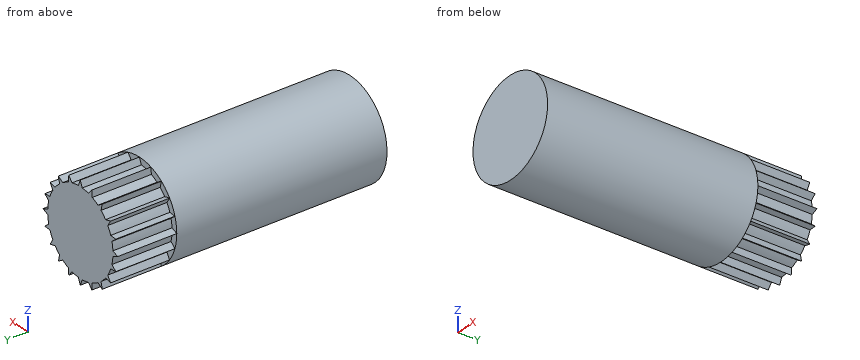
from build123d import *

# Parameters (mm, degrees)
SKETCH1_R           = 4.86
BOSS_EXTRUDE1_DEPTH = 21.336
BOSS_EXTRUDE2_DEPTH = 6


with BuildPart() as part:
    # Sketch1 → Boss-Extrude1 (new body)
    with BuildSketch(Plane(origin=(0, 0, 0), x_dir=(1, 0, 0), z_dir=(0, 1, 0))):
        with Locations(Location((0, 0, 0), (0, 0, 270))):
            Circle(SKETCH1_R)
    extrude(amount=BOSS_EXTRUDE1_DEPTH)

    # Sketch2 → Boss-Extrude2 (add)
    with BuildSketch(Plane(origin=(0, 21.336, 0), x_dir=(1, 0, 0), z_dir=(0, 1, 0))):
        with BuildLine():
            Line((0, 4.86), (0.250754017, 4.242596189))
            ThreePointArc((0.250754017, 4.242596189), (0.664846476, 4.197675448), (1.072553081, 4.112436004))
            Line((1.072553081, 4.112436004), (1.501822593, 4.622134669))
            Line((1.501822593, 4.622134669), (1.549515564, 3.957461499))
            ThreePointArc((1.549515564, 3.957461499), (1.929459624, 3.786777728), (2.29087121, 3.57972193))
            Line((2.29087121, 3.57972193), (2.856636326, 3.931822593))
            Line((2.856636326, 3.931822593), (2.696599732, 3.284942904))
            ThreePointArc((2.696599732, 3.284942904), (3.00520382, 3.00520382), (3.284942904, 2.696599732))
            Line((3.284942904, 2.696599732), (3.931822593, 2.856636326))
            Line((3.931822593, 2.856636326), (3.57972193, 2.29087121))
            ThreePointArc((3.57972193, 2.29087121), (3.786777728, 1.929459624), (3.957461499, 1.549515564))
            Line((3.957461499, 1.549515564), (4.622134669, 1.501822593))
            Line((4.622134669, 1.501822593), (4.112436004, 1.072553081))
            ThreePointArc((4.112436004, 1.072553081), (4.197675448, 0.664846476), (4.242596189, 0.250754017))
            Line((4.242596189, 0.250754017), (4.86, 0))
            Line((4.86, 0), (4.242596189, -0.250754017))
            ThreePointArc((4.242596189, -0.250754017), (4.197675448, -0.664846476), (4.112436004, -1.072553081))
            Line((4.112436004, -1.072553081), (4.622134669, -1.501822593))
            Line((4.622134669, -1.501822593), (3.957461499, -1.549515564))
            ThreePointArc((3.957461499, -1.549515564), (3.786777728, -1.929459624), (3.57972193, -2.29087121))
            Line((3.57972193, -2.29087121), (3.931822593, -2.856636326))
            Line((3.931822593, -2.856636326), (3.284942904, -2.696599732))
            ThreePointArc((3.284942904, -2.696599732), (3.00520382, -3.00520382), (2.696599732, -3.284942904))
            Line((2.696599732, -3.284942904), (2.856636326, -3.931822593))
            Line((2.856636326, -3.931822593), (2.29087121, -3.57972193))
            ThreePointArc((2.29087121, -3.57972193), (1.929459624, -3.786777728), (1.549515564, -3.957461499))
            Line((1.549515564, -3.957461499), (1.501822593, -4.622134669))
            Line((1.501822593, -4.622134669), (1.072553081, -4.112436004))
            ThreePointArc((1.072553081, -4.112436004), (0.664846476, -4.197675448), (0.250754017, -4.242596189))
            Line((0.250754017, -4.242596189), (0, -4.86))
            Line((0, -4.86), (-0.250754017, -4.242596189))
            ThreePointArc((-0.250754017, -4.242596189), (-0.664846476, -4.197675448), (-1.072553081, -4.112436004))
            Line((-1.072553081, -4.112436004), (-1.501822593, -4.622134669))
            Line((-1.501822593, -4.622134669), (-1.549515564, -3.957461499))
            ThreePointArc((-1.549515564, -3.957461499), (-1.929459624, -3.786777728), (-2.29087121, -3.57972193))
            Line((-2.29087121, -3.57972193), (-2.856636326, -3.931822593))
            Line((-2.856636326, -3.931822593), (-2.696599732, -3.284942904))
            ThreePointArc((-2.696599732, -3.284942904), (-3.00520382, -3.00520382), (-3.284942904, -2.696599732))
            Line((-3.284942904, -2.696599732), (-3.931822593, -2.856636326))
            Line((-3.931822593, -2.856636326), (-3.57972193, -2.29087121))
            ThreePointArc((-3.57972193, -2.29087121), (-3.786777728, -1.929459624), (-3.957461499, -1.549515564))
            Line((-3.957461499, -1.549515564), (-4.622134669, -1.501822593))
            Line((-4.622134669, -1.501822593), (-4.112436004, -1.072553081))
            ThreePointArc((-4.112436004, -1.072553081), (-4.197675448, -0.664846476), (-4.242596189, -0.250754017))
            Line((-4.242596189, -0.250754017), (-4.86, 0))
            Line((-4.86, 0), (-4.242596189, 0.250754017))
            ThreePointArc((-4.242596189, 0.250754017), (-4.197675448, 0.664846476), (-4.112436004, 1.072553081))
            Line((-4.112436004, 1.072553081), (-4.622134669, 1.501822593))
            Line((-4.622134669, 1.501822593), (-3.957461499, 1.549515564))
            ThreePointArc((-3.957461499, 1.549515564), (-3.786777728, 1.929459624), (-3.57972193, 2.29087121))
            Line((-3.57972193, 2.29087121), (-3.931822593, 2.856636326))
            Line((-3.931822593, 2.856636326), (-3.284942904, 2.696599732))
            ThreePointArc((-3.284942904, 2.696599732), (-3.00520382, 3.00520382), (-2.696599732, 3.284942904))
            Line((-2.696599732, 3.284942904), (-2.856636326, 3.931822593))
            Line((-2.856636326, 3.931822593), (-2.29087121, 3.57972193))
            ThreePointArc((-2.29087121, 3.57972193), (-1.929459624, 3.786777728), (-1.549515564, 3.957461499))
            Line((-1.549515564, 3.957461499), (-1.501822593, 4.622134669))
            Line((-1.501822593, 4.622134669), (-1.072553081, 4.112436004))
            ThreePointArc((-1.072553081, 4.112436004), (-0.664846476, 4.197675448), (-0.250754017, 4.242596189))
            Line((-0.250754017, 4.242596189), (0, 4.86))
        make_face()
    extrude(amount=BOSS_EXTRUDE2_DEPTH)


solid = part.part
Could you check a few things on this model? Use its own coordinates, in mm. Round coordinates to 2 decimals unless told otherwise and drop trailing zeros. Write each loop counter-clockwise with the first axis right and the second up, starting at its lowest first coordinate (ties: lowest second). Pieces come first, ordered by that corner, then holes. Notation, with made-up numbers: (7.25, 30) -> (46.25, 30) arc R8 cw to (46.25, 42) -> close; hole circle Ø8 at (16, 5). An arc over 180 degrees is marked (long way). Use a Markdown table: item, result.
1. If we section it at C-C (z = -0.5): List the corners of the cut face in (x, y) for me.
Answer key:
| item | result |
|---|---|
| outline | (-4.83, 0) -> (4.83, 0) -> (4.83, 21.34) -> (4.22, 21.34) -> (4.22, 27.34) -> (-4.22, 27.34) -> (-4.22, 21.34) -> (-4.83, 21.34) -> close |
2. If we section it at B-B (y = 13.25): List the corners of the cut face in (x, z) for me.
Answer key:
| item | result |
|---|---|
| outline | circle Ø9.72 at (0, 0) |
3. Please list where these lines run through material, in increasing order: probe 1 along X at (y, z) = (6.5, 0.25); probe 2 along Y at (x, z) = (-2, 4); probe 3 along Z at (x, y) = (1.75, 21.75).
Answer key:
| item | result |
|---|---|
| probe 1 | x = -4.85 to 4.85 |
| probe 2 | y = 0 to 21.34 |
| probe 3 | z = -3.87 to 3.87 |
4. If we section it at A-A (z = 0.75): List the corners of the cut face in (x, y) for me, then the cut area to 3 significant figures.
Answer key:
| item | result |
|---|---|
| outline | (-4.8, 0) -> (4.8, 0) -> (4.8, 21.34) -> (4.18, 21.34) -> (4.18, 27.34) -> (-4.18, 27.34) -> (-4.18, 21.34) -> (-4.8, 21.34) -> close |
| area | 255 mm^2 |
5. For pin 1 Ø1 at (y, z) = (6, -3.5) entering from +X; pin 2 Ø3 at (y, z) = (6.5, 3) entering from -X; pin 3 Ø1.5 at (x, z) = (3.5, -3) entering from -Y; pin 4 Ø0.8 at (x, z) = (4.5, 2) entering from +Y, each with a flat end and sliding along its axis, tell me the tip position at first contact or that it passes through.
Answer key:
| item | result |
|---|---|
| pin 1 | stops at x = 3.82 |
| pin 2 | stops at x = -4.62 |
| pin 3 | stops at y = 0 |
| pin 4 | stops at y = 21.34 |
